from build123d import *

# Parameters (mm, degrees)
F1_DEPTH = 2


with BuildPart() as f1:
    # F0 (on Top) → F1 (new body)
    with BuildSketch(Plane.XY):
        Polygon((302, 72.5), (275, 73.7069536424), (275, 0), (275, -73.7069536424), (302, -72.5), (302, 0), align=None)
        Polygon((0, 84), (0, 0), (0, -84), (0, -86), (275, -73.7069536424), (275, 0), (275, 73.7069536424), (0, 86), align=None)
        Polygon((0, -84), (0, 0), (0, 84), (-303, 67), (-303, 42), (-303, 0), (-303, -52), (-303, -67), align=None)
        Polygon((-2.8008756383, -133.9214893173), (0, -84), (-303, -67), (-304.7925604085, -98.9497531631), (-279.8318157498, -100.3501909822), (-280.7333549372, -118.3279178715), align=None)
        Polygon((-303, 67), (0, 84), (-2.8008756383, 133.9214893173), (-280.7333549372, 118.3279178715), (-279.8318157498, 100.3501909822), (-304.7925604085, 98.9497531631), align=None)
        Polygon((-303, 0), (-303, 42), (-353, 42), (-353, 0), (-353, -52), (-303, -52), align=None)
    extrude(amount=F1_DEPTH)


solid = f1.part
The listing builds one solid part. Answer for the finished solid, in the listing's coordinates (mm). Give positions to 0.01 mm unless a question says otherwise; leave off trailing zeros. Order: outer loops, then holes, each group sorted by start corner. A loop starts at its lowest first (then second) coordinate and runs counter-clockwise, first axis right, second up. Notation, with made-up numbers: (-10.75, 81) - (32.25, 81) arc R27 ccw to (32.25, 115) - close; hole circle Ø7 at (73.25, 71). An arc over 180 degrees is marked (long way). One line per item, written item: value. Start each with the question number.
1) A cutting plane is placed at C-C on x = -121. Give the vertices of the cut face in (y, z), then the cut area to 3 significant figures.
2) Given pin 1 Ø0.6 at (y, z) = (-85.5, 1) entering from -X; pin 2 Ø6 at (x, y) = (-134, 7.5) entering from -Z; pin 3 Ø1 at (y, z) = (58.5, 1) entering from -X, each flat-ended and moving along its own axis, determine where each tip first touches the part or whether it passes through.
3) A cutting plane is placed at B-B on x = 21.5. Give the vertices of the cut face in (y, z).
4) A cutting plane is placed at A-A on z = 0.65. Give the vertices of the cut face in (x, y), then the cut area to 3 significant figures.
5) Find the intervals of material crossed by L1, parallel to Y at x = -281, z = 0.6; L2, parallel to Y at x = -322.5, z = 1.1; L3, parallel to X at y = 66, z = 0.4, in increasing order.
Answer sheet:
1. outline: (-127.29, 0) - (127.29, 0) - (127.29, 2) - (-127.29, 2) - close
1. area: 509 mm2
2. pin 1: stops at x = -304.05
2. pin 2: stops at z = 0
2. pin 3: stops at x = -303
3. outline: (-85.04, 0) - (85.04, 0) - (85.04, 2) - (-85.04, 2) - close
4. outline: (-353, -52) - (-303, -52) - (-303, -67) - (-304.79, -98.95) - (-279.83, -100.35) - (-280.73, -118.33) - (-2.8, -133.92) - (0, -84) - (0, -86) - (302, -72.5) - (302, 72.5) - (0, 86) - (0, 84) - (-2.8, 133.92) - (-280.73, 118.33) - (-279.83, 100.35) - (-304.79, 98.95) - (-303, 67) - (-303, 42) - (-353, 42) - close
4. area: 128,000 mm2
5. L1: y = -100.28 to 100.28
5. L2: y = -52 to 42
5. L3: x = -303 to 302
